Geometry: final body of the model. Coordinates: model frame, mm. Face numbers are marked on the shaded views. A direction names the side the tool comes from. Round coordinates to 2 decimals unless told otherwise and drop trailing zeros. Loops run counter-clockwise (first coordinate to the right, second up) from the corner with the lowest first, then second, coordinate; pieces in that order, holes last. Notation, with made-up numbers: (4.5, -36) - (51.5, -36) arc R19 cw to (51.5, -26) - close; hole circle Ø7 at (48.5, 55.25). An arc over 180 degrees is marked (long way). Answer in a Markdown table with one row per item. Add a question column.
from build123d import *

# Parameters (mm, degrees)
ESQUISSE1_W          = 49.2
ESQUISSE1_H          = 52
BOSS_EXTRU_1_DEPTH   = 20
COQUE1_T             = 4
CONG_1_R             = 2
CONG_2_R             = 2
CONG_3_R             = 2
CONG_4_R             = 2
ESQUISSE5_R          = 1.8
BOSS_EXTRU_2_DEPTH   = 12
EMPREINTE1_START     = 9.306734089
EMPREINTE1_OUTLINE_W = 4
EMPREINTE1_OUTLINE_H = 6.8
EMPREINTE1_DEPTH     = 8


# Read off the part's stored shape, not the designer's step: Empreinte1
with BuildPart() as part:
    # Esquisse1 → Boss.-Extru.1 (new body)
    with BuildSketch(Plane(origin=(0, 0, 0), x_dir=(1, 0, 0), z_dir=(0, 1, 0))):
        Rectangle(ESQUISSE1_W, ESQUISSE1_H)
    extrude(amount=BOSS_EXTRU_1_DEPTH)

    # Coque1
    coque1_openings = [part.faces().sort_by_distance(p)[0] for p in [
        (0, 20, 0),
    ]]
    offset(amount=COQUE1_T, openings=coque1_openings, kind=Kind.INTERSECTION)

    # Congé1
    # the kernel refuses this fillet: 2 mm, written as the material it takes off along each edge
    with BuildSketch(Plane(origin=(28.6, -9, 30), x_dir=(-1, 0, 0), z_dir=(0, 1, 0))) as cong_1_piece_1:
        with BuildLine():
            CenterArc((CONG_1_R, -CONG_1_R), CONG_1_R, 90, 90)
            Line((0, -CONG_1_R), (0, 0))
            Line((0, 0), (CONG_1_R, 0))
        make_face()
    extrude(amount=34, mode=Mode.SUBTRACT)

    # Congé2
    cong_2_edges = [part.edges().sort_by_distance(p)[0] for p in [
        (28.6, 8, -30),
    ]]
    fillet(cong_2_edges, radius=CONG_2_R)

    # Congé3
    cong_3_edges = [part.edges().sort_by_distance(p)[0] for p in [
        (-28.6, 8, -30),
    ]]
    fillet(cong_3_edges, radius=CONG_3_R)

    # Congé4
    cong_4_edges = [part.edges().sort_by_distance(p)[0] for p in [
        (-28.6, 8, 30),
    ]]
    fillet(cong_4_edges, radius=CONG_4_R)

    # Esquisse5 → Boss.-Extru.2 (add)
    with BuildSketch(Plane(origin=(0, 0, 0), x_dir=(1, 0, 0), z_dir=(0, 1, 0))):
        with Locations(Location((-22.6, -2.6, 0), (0, 0, 90))):
            Circle(ESQUISSE5_R)
        with Locations(Location((22.6, -2.6, 0), (0, 0, 90))):
            Circle(ESQUISSE5_R)
        with Locations(Location((-22.6, -24, 0), (0, 0, 90))):
            Circle(ESQUISSE5_R)
        with Locations(Location((22.6, -24, 0), (0, 0, 90))):
            Circle(ESQUISSE5_R)
    extrude(amount=BOSS_EXTRU_2_DEPTH)

    # Empreinte1 outline → Empreinte1 (cut)
    with BuildSketch(Plane.XY.offset(EMPREINTE1_START)):
        with Locations((26.6, 16.6)):
            Rectangle(EMPREINTE1_OUTLINE_W, EMPREINTE1_OUTLINE_H)
    extrude(amount=EMPREINTE1_DEPTH, mode=Mode.SUBTRACT)


solid = part.part
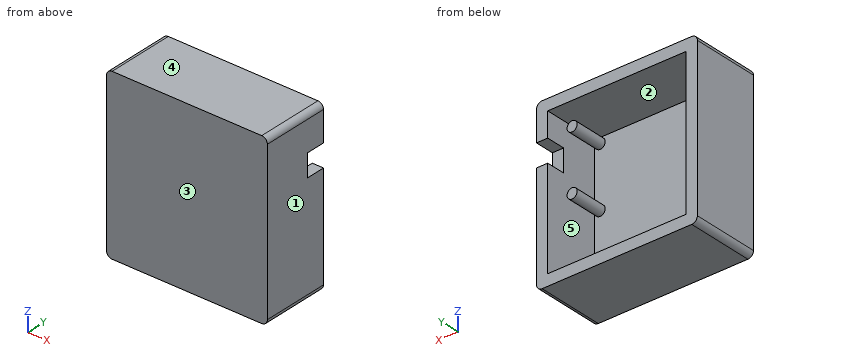
1) Section B-B, the plane z = 13.5. Return the cut outline in (x, y), and give its area (3 significant figures).
2) Section C-C, the plane x = -22.6. Return the cut outline in (y, z), and give its area (3 significant figures).
3) Pull-direction query (X, two-part tool) for the marked faces 1, 2 and 3; classes: pulls with the +X half, pulls with the -X half, needs draft (parallel to the pull), parting line crosses it, or undercut.
4) Material intervals for line 1 along Z through (x, y) = (7, 3.75); line 2 along X through (y, z) = (13, 14); line 3 along X through (y, z) = (3.5, 25.5), sorted ascending. Write a range as from..to.
5) Section A-A, the plane y = 4.5. Return the cut outline in (x, z).
6) Section D-D, the plane y = 14. Return the cut outline in (x, z), and give its area (3 significant figures).
7) Contact query for flat-ended pins moving along their axis: pin 1 Ø3 at (x, z) = (-21.5, 24) entering from +Y; pin 2 Ø1.2 at (x, y) = (27.5, 16) entering from +Z; pin 3 Ø3 at (x, z) = (26, 12) entering from +Y. Output: stop coordinate, or through.
8) Reachability of the marked faces 4 and 5 from +Z, -Z, +X, -X, +Y, -Y: full face, straight path, thin tool, end or side. Return the list, or none.
Evaluation:
| question | item | result |
|---|---|---|
| 1 | outline | (-28.6, -4) - (28.6, -4) - (28.6, 13.2) - (24.6, 13.2) - (24.6, 0) - (-24.6, 0) - (-24.6, 20) - (-28.6, 20) - close |
| 1 | area | 362 mm² |
| 2 | outline | (-4, -30) - (20, -30) - (20, -26) - (0, -26) - (0, 0.8) - (12, 0.8) - (12, 4.4) - (0, 4.4) - (0, 22.2) - (12, 22.2) - (12, 25.8) - (0, 25.8) - (0, 26) - (20, 26) - (20, 30) - (-4, 30) - close |
| 2 | area | 486 mm² |
| 3 | face 1 | pulls with the +X half |
| 3 | face 2 | undercut |
| 3 | face 3 | needs draft |
| 4 | line 1 | z = -30..-26, 26..30 |
| 4 | line 2 | x = -28.6..-24.6, 24.6..28.6 |
| 4 | line 3 | x = -28.6..-24.6, -23.59..-21.61, 21.61..23.59, 24.6..28.6 |
| 5 | outline | (-28.6, -28) arc R2 ccw to (-26.6, -30) - (26.6, -30) arc R2 ccw to (28.6, -28) - (28.6, 28) arc R2 ccw to (26.6, 30) - (-26.6, 30) arc R2 ccw to (-28.6, 28) - close; circle Ø3.6 at (-22.6, 2.6); circle Ø3.6 at (-22.6, 24); circle Ø3.6 at (22.6, 2.6); circle Ø3.6 at (22.6, 24); hole (-24.6, -26) - (24.6, -26) - (24.6, 26) - (-24.6, 26) - close |
| 6 | outline | (-28.6, -28) arc R2 ccw to (-26.6, -30) - (26.6, -30) arc R2 ccw to (28.6, -28) - (28.6, 9.31) - (24.6, 9.31) - (24.6, -26) - (-24.6, -26) - (-24.6, 26) - (24.6, 26) - (24.6, 17.31) - (28.6, 17.31) - (28.6, 28) arc R2 ccw to (26.6, 30) - (-26.6, 30) arc R2 ccw to (-28.6, 28) - close |
| 6 | area | 838 mm² |
| 7 | pin 1 | stops at y = 12 |
| 7 | pin 2 | stops at z = 29.98 |
| 7 | pin 3 | stops at y = 13.2 |
| 8 | face 4 | +Z, +X, -X, +Y, -Y |
| 8 | face 5 | +Y |
